The drawing under review shows one solid part. Ordinate dimensions are in mm from its lowest x, y, z. A direction names the side the tool comes from. Round coordinates to 2 decimals unless told otherwise and drop trailing zeros. Order: outer loops, then holes, each group sorted by start corner. A loop starts at its lowest first (then second) coordinate and runs counter-clockwise, first axis right, second up.
1) Consider section D-D (x = 57.15). Give the boundary of the cut face in (y, z).
2) Consider section C-C (z = 14.5). Give the boundary of the cut face in (x, y), then the cut area to 3 significant figures.
3) Clearance check with flat-ended pins moving along their axes: P1, Ø1, axis at x = 58, y = 91, coming from the -Z side; P2, Ø11.5, axis at x = 55, y = 42, coming from the +Z side; P3, Ø6, axis at x = 77.5, z = 48, coming from the -Y side. State where each tip first meets the part, or that it passes through.
4) To check wall thickness, follow L1, parallel to X at y = 79.5, z = 66; L2, parallel to X at y = 58, z = 22; L3, parallel to Z at x = 38, y = 16. State the ranges of each line that lie inside material, in increasing order.
5) Machinability: for the marked faces 1 and 2, which of the approach directions +Z, -Z, +X, -X, +Y, -Y give a long, thin tool a straight path to every point of the face, cutting with its end or side? Answer none if there is none.
6) Consider section A-A (z = 73). Give the boundary of the cut face in (x, y), then the cut area to 3 significant figures.
7) Consider section B-B (y = 61). Give the boundary of the cut face in (x, z), then the cut area to 3 significant figures.
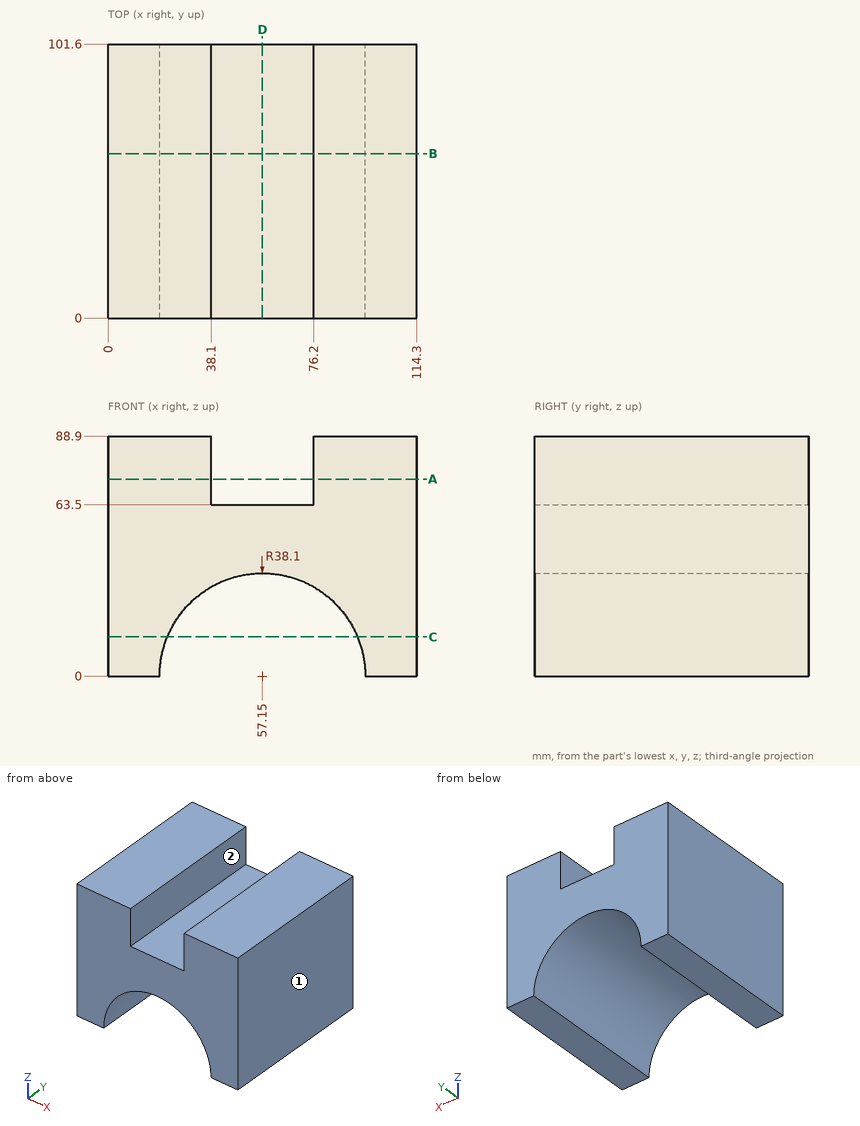
Answer below:
1. outline: (0, 38.1) - (101.6, 38.1) - (101.6, 63.5) - (0, 63.5) - close
2. outline: (0, 0) - (21.92, 0) - (21.92, 101.6) - (0, 101.6) - close; (92.38, 0) - (114.3, 0) - (114.3, 101.6) - (92.38, 101.6) - close
2. area: 4,450 mm2
3. P1: stops at z = 38.08
3. P2: stops at z = 63.5
3. P3: stops at y = 0
4. L1: x = 0 to 38.1, 76.2 to 114.3
4. L2: x = 0 to 26.04, 88.26 to 114.3
4. L3: z = 32.94 to 88.9
5. face 1: +Z, -Z, +X, +Y, -Y
5. face 2: +Z, +Y, -Y
6. outline: (0, 0) - (38.1, 0) - (38.1, 101.6) - (0, 101.6) - close; (76.2, 0) - (114.3, 0) - (114.3, 101.6) - (76.2, 101.6) - close
6. area: 7,740 mm2
7. outline: (0, 0) - (19.05, 0) arc R38.1 cw to (95.25, 0) - (114.3, 0) - (114.3, 88.9) - (76.2, 88.9) - (76.2, 63.5) - (38.1, 63.5) - (38.1, 88.9) - (0, 88.9) - close
7. area: 6,910 mm2
